Geometry check sheet. Reference: the model listing, model coordinates, mm. Face numbers are marked on the shaded views. Round coordinates to 2 decimals unless told otherwise and drop trailing zeros. Write each loop counter-clockwise with the first axis right and the second up, starting at its lowest first coordinate (ties: lowest second). Pieces come first, ordered by that corner, then holes.
Item 1: Cross-section at D-D (y = 8.75). Enter the section's corners in (x, z), then the cut area to 3 significant figures.
Item 2: Depth check by flat-ended pin: P1, Ø1.5, axis at x = 1.5, y = 1, coming from the +Z side; P2, Ø5, axis at y = 3.5, z = 5, coming from the -X side; P3, Ø1, axis at y = 7.5, z = 2.5, coming from the -X side. Enter the tip coordinate at first touch or a pass-through.
Item 3: Draft check along Z on the marked faces 1, 2, 3 and 4. Enter one of: pulls with the +Z half, pulls with the -Z half, needs draft (parallel to the pull), parting line crosses it, or undercut.
Item 4: Cross-section at A-A (x = 0). Enter the section's corners in (y, z), then the cut area to 3 significant figures.
Item 5: Scan lines: probe 1 along X at (y, z) = (2, 0); probe 2 along X at (y, z) = (12.25, 0); probe 3 along Z at (x, y) = (1.5, -7.5). Record each from-to range of solid material in increasing order.
Item 6: Cross-section at C-C (y = 3). Enter the section's corners in (x, z).
Item 7: Cross-section at B-B (z = 0). Enter the section's corners in (x, y).
from build123d import *

# Parameters (mm, degrees)
CORTAR_EXTRUIR1_START = -13
CROQUIS3_R            = 7
CROQUIS3_R_2          = 3.134205676
CORTAR_EXTRUIR1_DEPTH = 13


with BuildPart() as part:
    # Croquis1 → Revolución1 (revolve)
    with BuildSketch(Plane.XY, mode=Mode.PRIVATE) as revoluci_n1_sk:
        with BuildLine():
            Line((-3.134205676, -13), (-6.134205676, -13))
            ThreePointArc((-6.134205676, -13), (-9.669739582, -11.535533906), (-11.134205676, -8))
            Line((-11.134205676, -8), (-11.134205676, 8))
            ThreePointArc((-11.134205676, 8), (-9.669739582, 11.535533906), (-6.134205676, 13))
            Line((-6.134205676, 13), (-3.134205676, 13))
            Line((-3.134205676, 13), (-3.134205676, -13))
        make_face()
    revolve(revoluci_n1_sk.sketch.rotate(Axis((0, 13, 0), (0, -1, 0)), 270), axis=Axis((0, 13, 0), (0, -1, 0)))

    # Croquis3 → Cortar-Extruir1 (cut)
    with BuildSketch(Plane(origin=(0, 23, 0), x_dir=(1, 0, 0), z_dir=(0, 1, 0)).offset(CORTAR_EXTRUIR1_START)):
        with Locations(Location((0, 0, 0), (0, 0, 270))):
            Circle(CROQUIS3_R)
        with Locations(Location((0, 0, 0), (0, 0, 270))):
            Circle(CROQUIS3_R_2, mode=Mode.SUBTRACT)
    extrude(amount=CORTAR_EXTRUIR1_DEPTH, mode=Mode.SUBTRACT)


solid = part.part
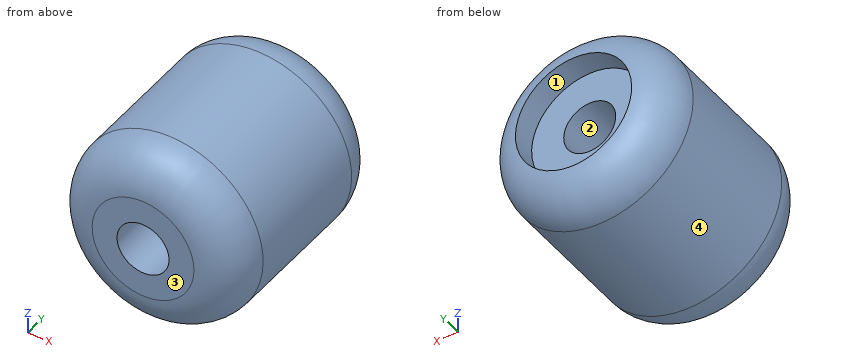
Resolved:
1. outline: circle Ø22.16 at (0, 0); hole circle Ø6.27 at (0, 0)
1. area: 355 mm2
2. P1: stops at z = 11.11
2. P2: stops at x = -10.85
2. P3: stops at x = -10.95
3. face 1: undercut
3. face 2: undercut
3. face 3: needs draft
3. face 4: parting line crosses it
4. outline: (-13, -6.13) arc R5 ccw to (-8, -11.13) - (8, -11.13) arc R5 ccw to (12.92, -7) - (10, -7) - (10, -3.13) - (-13, -3.13) - close; (-13, 3.13) - (10, 3.13) - (10, 7) - (12.92, 7) arc R5 ccw to (8, 11.13) - (-8, 11.13) arc R5 ccw to (-13, 6.13) - close
4. area: 371 mm2
5. probe 1: x = -11.13 to -3.13, 3.13 to 11.13
5. probe 2: x = -8.77 to -7, 7 to 8.77
5. probe 3: z = -11.03 to -2.75, 2.75 to 11.03
6. outline: circle Ø22.27 at (0, 0); hole circle Ø6.27 at (0, 0)
7. outline: (-11.13, -8) arc R5 ccw to (-6.13, -13) - (-3.13, -13) - (-3.13, 10) - (-7, 10) - (-7, 12.92) arc R5 ccw to (-11.13, 8) - close; (3.13, -13) - (6.13, -13) arc R5 ccw to (11.13, -8) - (11.13, 8) arc R5 ccw to (7, 12.92) - (7, 10) - (3.13, 10) - close
